Can you work these out from the model? Positions are in its coordinate system, mm. A direction names the side the tool comes from. Round coordinates to 2 decimals unless told otherwise and drop trailing zeros. Loops run counter-clockwise (first coordinate to the right, second up) from the corner with the lowest first, then second, coordinate; pieces in that order, holes last.
(1) If I drill on line 1 along X through (y, z) = (2, -1.75); line 2 along Y through (x, z) = (-2.5, -0.75); line 3 along Y through (x, z) = (18.5, -1), over which ranges is the centre line in solid material (lowest first)?
(2) Which directions (+Z, -Z, +X, -X, +Y, -Y) give clear straight access to the entire face, cutting with the end or side of a thin tool? Please do faces 1 (the face through (-2.948, 0.74, -1.305)), 2 (the face through (10, 0, 2)), 3 (the face through (20, 0, 0)).
(3) I want a section at A-A on x = 5. Write out the boundary of the cut face in (y, z).
(4) Thinking about a two-plate mould opening in Z: for faces 4 (the face through (-1.825, 3.233, 1.341)), 5 (the face through (-3, 1.5, 0)), 6 (the face through (-4, -1.3, 1.3)), which applies, released by +Z, released by -Z, zero draft, split by the parting line, or undercut?
(5) Will these pins go through, and if not, where does the flat tip stop? pin 1 Ø3 at (x, y) = (0.5, -2) entering from -Z; pin 2 Ø3 at (x, y) = (0, 2) entering from -Z; pin 3 Ø2 at (x, z) = (7.5, -0.5) entering from -Y.
Autodesk Inventor part; units mm, degrees
ref_plane "Work Plane1" through (29, 0, 0) normal (0, -1, 0) x (1, 0, 0)
ref_plane "YZ Plane" through (0, 0, 0) normal (1, 0, 0) x (0, 1, 0)
ref_plane "XZ Plane" through (0, 0, 0) normal (0, 1, 0) x (-1, 0, 0)
sketch "Skizze1" plane through (0, 0, 0) normal (0, 0, 1) x (1, 0, 0)
  line L0 (-1, 0) -> (20, 0)
  line L1 (20, 0) -> (20, 2)
  line L2 (20, 2) -> (1.75, 2)
  line L3 (1.75, 2) -> (1.3205, 2)
  line L4 (1.3205, 2) -> (0, 2)
  line L5 (0, 2) -> (0, 3.5)
  line L6 (0, 3.5) -> (-4, 3.5)
  line L7 (-4, 3.5) -> (-4, 1.7321)
  line L8 (-4, 1.7321) -> (-2, 1.7321)
  line L9 (-2, 1.7321) -> (-1, 0)
  line L10 (-8.8, 0) -> (24.8, 0)
  line L11 (0, -0.7) -> (0, 4.2)
  line L12 (1.75, 2) -> (0, 2) construction
  dimension "d1" = 18.25
  dimension "d2" = 0.4295
  dimension "d3" = 4
  dimension "d4" = 2
  dimension "d5" = 60
  dimension "d6" = 4
  dimension "d7" = 4
  dimension "d8" = 3.4641
  dimension "d9" = 7
  dimension "d26" = 20
revolve "Körper" add sketch "Skizze1" angle 360 about axis through (-1, 0, 0) along (1, 0, 0)
sketch "Skizze2" plane through (-4, 0, 0) normal (-1, 0, 0) x (0, 0, 1)
  circle A0 centre (0, 0) radius 1.7321
  line L0 (0, -4.9) -> (0, 4.9)
  line L1 (-4.9, 0) -> (4.9, 0)
  line L2 (1.7321, 0) -> (0.866, -1.5)
  line L3 (0.866, -1.5) -> (-0.866, -1.5)
  line L4 (-0.866, -1.5) -> (-1.7321, 0)
  line L5 (-1.7321, 0) -> (-0.866, 1.5)
  line L6 (-0.866, 1.5) -> (0.866, 1.5)
  line L7 (0.866, 1.5) -> (1.7321, 0)
extrude "Loch" add sketch "Skizze2" against normal up to next contours L7 A0 | A0 L2 | L6 L0 A0 | A0 L0 L3 | L0 L6 A0 | A0 L3 L0 | L4 A0 | A0 L5
fillet "Rundung1" radius 0.4 1 edges at (-4, -3.5, 0)
thread "Gewinde"
chamfer "Fase1" distance 0.4294 distance2 0.4294 1 edges at (20, -2, 0) measured on face at (20, 0.0679, 1.2634)
ref_plane "Work Plane1" through (29, 0, 0) normal (0, -1, 0) x (1, 0, 0)
fillet "Fillet2" radius 0.2 1 edges at (0, -2, 0)
equation "\"d1\" = GEL"
equation "\"d3\" = KOH"
equation "\"d4\" = INTI"
equation "\"d6\" = GD"
equation "\"d7\" = BDM"
equation "\"d8\" = 1.1547 * SW"
equation "\"d9\" = KOD"
equation "\"d26\" = NLG"
equation "\"d30\" = R"
equation "\"d17\" = RR"
equation "\"d13\" = GEL"
equation "\"d15\" = -0.5 * SPD + 0.5 * GD"
equation "\"d16\" = GUL"
equation "\"GD\" = NND"
equation "\"NLG\" = 20"
equation "\"GEL\" = 18.25"
equation "\"KOD\" = 7"
equation "\"KOH\" = 4"
equation "\"INTI\" = 2"
equation "\"GAL\" = 0.61345 * PTC"
equation "\"GUL\" = 0.61345 * PTC"
equation "\"BDM\" = NND"
equation "\"SW\" = 3"
equation "\"RR\" = 0.4"
equation "\"SPD\" = NND - 1.2269 * PTC"
equation "\"R\" = 0.2"
equation "\"TOA\" = 30deg"
equation "\"GD1\" = THREADDIA - 1.2269 * PTC"
equation "\"THREADDIA\" = 4"
equation "\"FAWI\" = 45deg"
equation "\"ANG\" = 120deg"
equation "\"PTC\" = 0.7"
equation "\"NND\" = 4"
equation "\"E0\" = 1.155 * SW"
properties part number "DIN 912 - M4 x 20" material "Stahl, weich"
Filled sheet:
1. line 1: x = -4 to 0
1. line 2: y = -3.42 to -1.5, 1.5 to 3.42
1. line 3: y = -1.73 to 1.73
2. face 1: -X
2. face 2: +X
2. face 3: +Z, -Z, +X, +Y, -Y
3. outline: circle Ø4 at (0, 0)
4. face 4: split by the parting line
4. face 5: undercut
4. face 6: zero draft
5. pin 1: stops at z = -3.45
5. pin 2: stops at z = -3.46
5. pin 3: stops at y = -2
